Could you check a few things on this model? Use its own coordinates, in mm. A direction names the side the tool comes from. Coordinates: 2 decimals unless noted, no trailing zeros. Order: outer loops, then holes, each group sorted by start corner. A loop starts at its lowest first (then second) coordinate and runs counter-clockwise, first axis right, second up. Notation, with made-up numbers: (23.25, -32) - (82.25, -32) arc R13 ccw to (82.25, -12) - close; hole circle Ø8 at (-20, 36.5). An arc over 180 degrees is marked (long way). One line per item, written item: value.
Autodesk Inventor part; units mm, degrees
ref_plane "YZ Plane" through (0, 0, 0) normal (1, 0, 0) x (0, 1, 0)
ref_plane "XZ Plane" through (0, 0, 0) normal (0, 1, 0) x (-1, 0, 0)
ref_plane "XY Plane" through (0, 0, 0) normal (0, 0, 1) x (1, 0, 0)
sketch "スケッチ1" plane through (0, 0, 0) normal (0, 0, 1) x (1, 0, 0)
  circle A0 centre (0, 0) radius 3
  dimension "d0" = 6
extrude "押し出し1" add sketch "スケッチ1" along normal blind 25
hole "穴1" at (0, 0, 0) direction (0, 0, 1) diameter 3 depth 6 tip angle 118
sketch "スケッチ2" plane through (0, 0, 25) normal (0, 0, 1) x (1, 0, 0)
  circle A0 centre (0, 0) radius 3
hole "穴2" at (0, 0, 25) direction (0, 0, -1) diameter 3 depth 6 tip angle 118
properties part number "スペーサ　m3-l25" material "アルミニウム 2014-T4"
Item 1: If I drill on probe 1 along Y at (x, z) = (0, 21.2); probe 2 along Y at (x, z) = (-2.6, 5); probe 3 along Y at (x, z) = (0.7, 23.5), over which ranges is the centre line in solid material (lowest first)?
Conclusion:
probe 1: -3 to -1.5, 1.5 to 3
probe 2: -1.5 to 1.5
probe 3: -2.92 to -1.33, 1.33 to 2.92
Item 2: For faces 1 (the face through (-0.07, 1.5, 21.96)), 2 (the face through (1.3, -1.3, 0)), which set-ups out of +Z, -Z, +X, -X, +Y, -Y let a thin tool reach every point of the face, with its end or its side?
Conclusion:
face 1: +Z
face 2: -Z, +X, -X, +Y, -Y
Item 3: I'm going to push flat-ended pins straight in: pin 1 Ø1 at (y, z) = (-1, 10.5) entering from +X; pin 2 Ø1.8 at (x, y) = (0, 0) entering from -Z. Where does each tip first touch, or does it pass through?
Conclusion:
pin 1: x = 2.96
pin 2: z = 6.36
Item 4: I want a section at B-B on y = 1.8. Please give me the cut outline in (x, z).
Conclusion:
outline: (-2.4, 0) - (2.4, 0) - (2.4, 25) - (-2.4, 25) - close
Item 5: Thinking about a two-plate mould opening in Y: for faces 3 (the face through (-0.07, -1.5, 3.04)), 4 (the face through (1.3, -1.3, 25)), 5 (the face through (-3, 0, 12)), which applies, pulls with the +Y half, pulls with the -Y half, needs draft (parallel to the pull), parting line crosses it, or undercut?
Conclusion:
face 3: undercut
face 4: needs draft
face 5: parting line crosses it
Item 6: I want a section at A-A on z = 21.5. Please give me the cut outline in (x, y).
Conclusion:
outline: circle Ø6 at (0, 0); hole circle Ø3 at (0, 0)
Item 7: I want a section at D-D on x = -2.15. Please give me the cut outline in (y, z).
Conclusion:
outline: (-2.09, 0) - (2.09, 0) - (2.09, 25) - (-2.09, 25) - close
Item 8: I want a section at C-C on z = 8. Please give me the cut outline in (x, y).
Conclusion:
outline: circle Ø6 at (0, 0)
